```python
from build123d import *

# Parameters (mm, degrees)
SKETCH1_W           = 28
SKETCH1_H           = 30
BOSS_EXTRUDE1_DEPTH = 3
SKETCH2_R           = 1.6
CUT_EXTRUDE1_DEPTH  = 4
SKETCH3_W           = 28
SKETCH3_H           = 17
CUT_EXTRUDE2_DEPTH  = 4
FILLET1_R           = 2


with BuildPart() as part:
    # Sketch1 → Boss-Extrude1 (new body)
    with BuildSketch(Plane(origin=(0, 0, 0), x_dir=(1, 0, 0), z_dir=(0, 1, 0))):
        Rectangle(SKETCH1_W, SKETCH1_H)
        with BuildLine():
            ThreePointArc((1.5, 8.4), (0.687397597, 8.621712173), (0.1, 9.225403331))
            Line((0.1, 9.225403331), (0.1, 5))
            ThreePointArc((0.1, 5), (-1.5, 3.4), (-3.1, 5))
            Line((-3.1, 5), (-3.1, 8.4))
            Line((-3.1, 8.4), (-6.5, 8.4))
            ThreePointArc((-6.5, 8.4), (-8.1, 10), (-6.5, 11.6))
            Line((-6.5, 11.6), (-1.5, 11.6))
            ThreePointArc((-1.5, 11.6), (-0.586447127, 11.313552873), (0, 10.556776436))
            ThreePointArc((0, 10.556776436), (0.586447127, 11.313552873), (1.5, 11.6))
            Line((1.5, 11.6), (6.5, 11.6))
            ThreePointArc((6.5, 11.6), (7.63137085, 11.13137085), (8.1, 10))
            Line((8.1, 10), (8.1, 5))
            ThreePointArc((8.1, 5), (6.5, 3.4), (4.9, 5))
            Line((4.9, 5), (4.9, 8.4))
            Line((4.9, 8.4), (1.5, 8.4))
        make_face(mode=Mode.SUBTRACT)
    extrude(amount=BOSS_EXTRUDE1_DEPTH)

    # Sketch2 → Cut-Extrude1 (cut, through all)
    with BuildSketch(Plane(origin=(0, 3, 0), x_dir=(1, 0, 0), z_dir=(0, 1, 0))):
        with Locations((-5.25, -10)):
            Circle(SKETCH2_R)
        with Locations((5.25, -10)):
            Circle(SKETCH2_R)
        Polygon((14, 0), (8.5, -15), (14, -15), align=None)
        Polygon((-8.5, -15), (-14, -15), (-14, 0), align=None)
    extrude(amount=-CUT_EXTRUDE1_DEPTH, mode=Mode.SUBTRACT)

    # Sketch3 → Cut-Extrude2 (cut, through all)
    with BuildSketch(Plane(origin=(0, 3, 0), x_dir=(1, 0, 0), z_dir=(0, 1, 0))):
        with Locations((0, -6.5)):
            Rectangle(SKETCH3_W, SKETCH3_H)
    extrude(amount=-CUT_EXTRUDE2_DEPTH, mode=Mode.SUBTRACT)

    # Fillet1
    fillet1_edges = [part.edges().sort_by_distance(p)[0] for p in [
        (-14, 1.5, -15),
        (14, 1.5, -15),
        (14, 1.5, -2),
        (-14, 1.5, -2),
    ]]
    fillet(fillet1_edges, radius=FILLET1_R)


solid = part.part
```
Design review of the part built by this model. Coordinates are the model's own, in mm. A direction names the side the tool comes from. Coordinates: 2 decimals unless noted, no trailing zeros. Order: outer loops, then holes, each group sorted by start corner. A loop starts at its lowest first (then second) coordinate and runs counter-clockwise, first axis right, second up. Notation, with made-up numbers: (11, 10) - (37, 10) arc R14 ccw to (37, 30) - close; hole circle Ø1 at (-28.75, -26.75). An arc over 180 degrees is marked (long way). Answer in a Markdown table with one row per item.
(1) Wall thickness on line 1 along Z through (x, y) = (-2.75, 1.2); line 2 along Z through (x, y) = (1.5, 0.7); line 3 along X through (y, z) = (2.45, -7): over which ranges is each line inside the solid? List them lowest first. Write a range as from..to.
Checked values:
| item | result |
|---|---|
| line 1 | -15..-11.6, -4..-2 |
| line 2 | -15..-11.6, -8.4..-2 |
| line 3 | -14..-3.1, 0.1..4.9, 8.1..14 |
(2) For faces 4 (the cylindrical face through (6.5, 1.5, -3.4)), 5 (the flat face through (-14, 1, -8)), list the 3-axis set-ups (+Z, -Z, +X, -X, +Y, -Y) from which the entire face can be reached by the end or side of a thin tool; tool diameter is ignored.
Checked values:
| item | result |
|---|---|
| face 4 | +Y, -Y |
| face 5 | +Z, -Z, -X, +Y, -Y |
(3) The part is to be moulded in two halves that separate along Z. For faces 1 (the cylindrical face through (13.4, 1.48, -2.57)), 2 (the flat face through (14, 1, -8)), 3 (the flat face through (3, 1, -8.4)), say which applies: released by +Z, released by -Z, zero draft, split by the parting line, or undercut.
Checked values:
| item | result |
|---|---|
| face 1 | released by +Z |
| face 2 | zero draft |
| face 3 | undercut |
(4) Consider section B-B on y = 0.8. State the section outline as (x, z) points, plus the area to 3 significant figures.
Checked values:
| item | result |
|---|---|
| outline | (-14, -13) arc R2 ccw to (-12, -15) - (12, -15) arc R2 ccw to (14, -13) - (14, -4) arc R2 ccw to (12, -2) - (-12, -2) arc R2 ccw to (-14, -4) - close; hole (-6.5, -11.6) - (-1.5, -11.6) arc R1.6 ccw to (0, -10.56) arc R1.6 ccw to (1.5, -11.6) - (6.5, -11.6) arc R1.6 ccw to (8.1, -10) - (8.1, -5) arc R1.6 ccw to (4.9, -5) - (4.9, -8.4) - (1.5, -8.4) arc R1.6 ccw to (0.1, -9.23) - (0.1, -5) arc R1.6 ccw to (-3.1, -5) - (-3.1, -8.4) - (-6.5, -8.4) arc R1.6 ccw to start |
| area | 282 mm^2 |
(5) Consider section A-A on z = -5.5. State the section outline as (x, y) points, plus the area to 3 significant figures.
Checked values:
| item | result |
|---|---|
| outline | (-14, 0) - (-3.1, 0) - (-3.1, 3) - (-14, 3) - close; (0.1, 0) - (4.9, 0) - (4.9, 3) - (0.1, 3) - close; (8.1, 0) - (14, 0) - (14, 3) - (8.1, 3) - close |
| area | 64.8 mm^2 |
